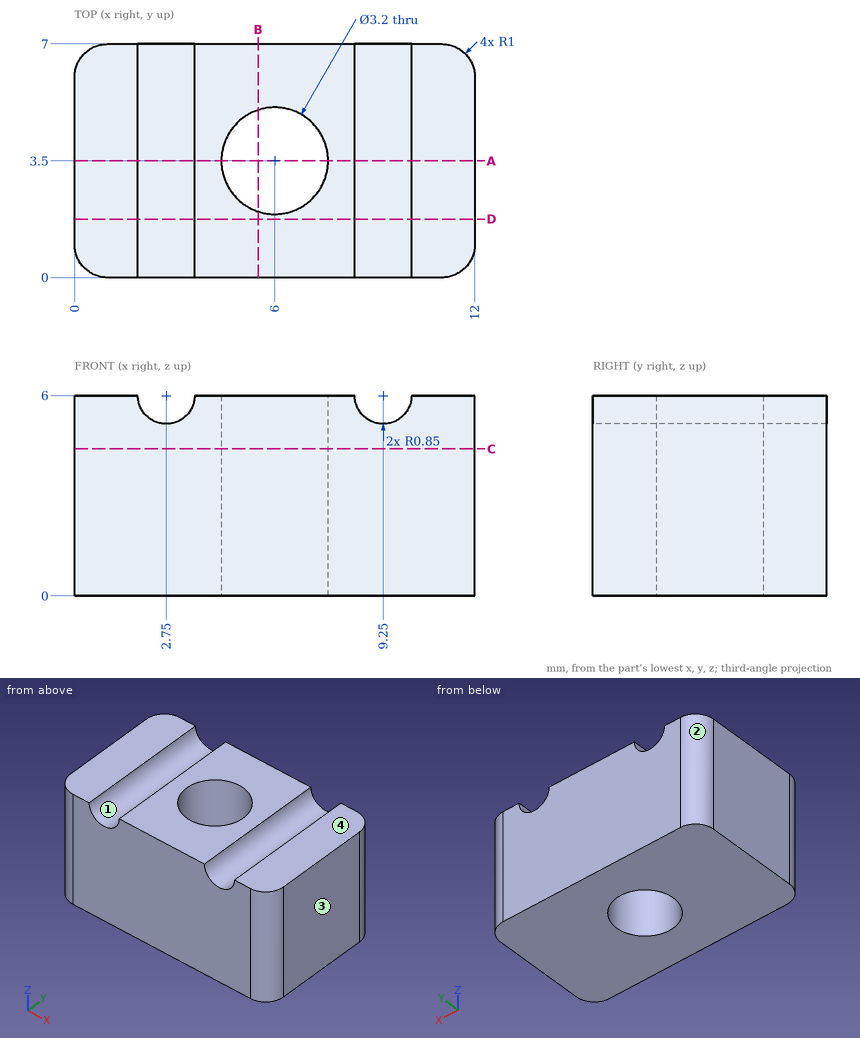
Here's the drawing with two shaded views (mm, measured from the low corner). I have some questions. Give positions to 0.01 mm unless a question says otherwise; leave off trailing zeros. Order: outer loops, then holes, each group sorted by start corner. A loop starts at its lowest first (then second) coordinate and runs counter-clockwise, first axis right, second up. Notation, with made-up numbers: (62, -34.5) -> (106, -34.5) arc R31 ccw to (106, -5.5) -> close; hole circle Ø11 at (88, -1.5). An arc over 180 degrees is marked (long way). Use a Markdown table: item, result. Add a question column.
Item 1: I need wall thicknesses on line 1 (Y direction, x = 6, z = 1.9); line 2 (X direction, y = 6, z = 5.75); line 3 (Y direction, x = 5, z = 4.65). Which ranges of each line are inside material? Lowest first, please.
Item 2: Imagine slicing it at B-B on x = 5.5. Please give me the cut outline in (y, z), plus the area to 3 significant figures.
Item 3: Imagine slicing it at A-A on y = 3.5. Please give me the cut outline in (x, z), plus the area to 3 significant figures.
Item 4: Imagine slicing it at C-C on z = 4.4. Please give me the cut outline in (x, y).
Item 5: Imagine slicing it at D-D on y = 1.75. Please give me the cut outline in (x, z), plus the area to 3 significant figures.
Item 6: Will this pin go through, and if not, where does the flat tip stop? pin 1 (4 mm diameter, centred on x = 8.5, y = 5.5, fed in from -Z).
Item 7: If we mould it in two halves opening along X, with no side actions, what happens to the marked faces 1, 2, 3 and 4? For each: pulls with the +X half, pulls with the -X half, needs draft (parallel to the pull), parting line crosses it, or undercut.
Data:
| question | item | result |
|---|---|---|
| 1 | line 1 | y = 0 to 1.9, 5.1 to 7 |
| 1 | line 2 | x = 0 to 1.94, 3.56 to 8.44, 10.06 to 12 |
| 1 | line 3 | y = 0 to 2.25, 4.75 to 7 |
| 2 | outline | (0, 0) -> (1.98, 0) -> (1.98, 6) -> (0, 6) -> close; (5.02, 0) -> (7, 0) -> (7, 6) -> (5.02, 6) -> close |
| 2 | area | 23.8 mm² |
| 3 | outline | (0, 0) -> (4.4, 0) -> (4.4, 6) -> (3.6, 6) arc R0.85 cw to (1.9, 6) -> (0, 6) -> close; (7.6, 0) -> (12, 0) -> (12, 6) -> (10.1, 6) arc R0.85 cw to (8.4, 6) -> (7.6, 6) -> close |
| 3 | area | 50.5 mm² |
| 4 | outline | (0, 1) arc R1 ccw to (1, 0) -> (11, 0) arc R1 ccw to (12, 1) -> (12, 6) arc R1 ccw to (11, 7) -> (1, 7) arc R1 ccw to (0, 6) -> close; hole circle Ø3.2 at (6, 3.5) |
| 5 | outline | (0, 0) -> (12, 0) -> (12, 6) -> (10.1, 6) arc R0.85 cw to (8.4, 6) -> (3.6, 6) arc R0.85 cw to (1.9, 6) -> (0, 6) -> close |
| 5 | area | 69.7 mm² |
| 6 | pin 1 | stops at z = 0 |
| 7 | face 1 | undercut |
| 7 | face 2 | pulls with the -X half |
| 7 | face 3 | pulls with the +X half |
| 7 | face 4 | needs draft |
